from build123d import *

# Parameters (mm, degrees)
SKETCH_W           = 33
SKETCH_H           = 14
PAD_DEPTH          = 38
SKETCH001_W        = 4
SKETCH001_H        = 58.5
PAD001_DEPTH       = 33
SKETCH002_W        = 10
SKETCH002_H        = 4
PAD002_DEPTH       = 33
SKETCH003_W        = 32
SKETCH003_H        = 5
SKETCH003_H_2      = 9
SKETCH003_H_3      = 14
POCKET_DEPTH       = 12
POCKET_FACE14_W    = 33
POCKET_FACE14_H    = 38
POCKET_FACE14_W_2  = 32
POCKET_FACE14_H_2  = 5
POCKET_FACE14_H_3  = 9
POCKET_FACE14_H_4  = 14
POCKET001_DEPTH    = 2
SKETCH004_W        = 33
SKETCH004_H        = 38
SKETCH004_W_2      = 32
SKETCH004_H_2      = 4
SKETCH004_H_3      = 8
SKETCH004_H_4      = 13
PAD003_DEPTH       = 2
POCKET002_DEPTH    = 1
POCKET003_DEPTH    = 31.5
SKETCH006_W        = 14
SKETCH006_H        = 38
PAD004_DEPTH       = 1
PAD005_DEPTH       = 1
SKETCH007_W        = 37
SKETCH007_H        = 14
PAD006_DEPTH       = 2
SKETCH008_W        = 37
SKETCH008_H        = 2
PAD007_DEPTH       = 4
FILLET_R           = 4.74
FILLET001_R        = 4.74
FILLET002_R        = 1
FILLET003_R        = 1
FILLET004_R        = 1
FILLET005_R        = 1
FILLET005_FACE22_W = 18
FILLET005_FACE22_H = 2
PAD008_DEPTH       = 2
PAD008_FACE3_W     = 14
PAD008_FACE3_H     = 38
PAD009_DEPTH       = 2
PAD009_FACE3_W     = 18
PAD009_FACE3_H     = 2
PAD010_DEPTH       = 2
PAD010_FACE1_W     = 14
PAD010_FACE1_H     = 38
PAD011_DEPTH       = 2
SKETCH009_W        = 20
SKETCH009_H        = 11
POCKET004_DEPTH    = 38
FILLET006_R        = 5
FILLET007_R        = 1
FILLET008_R        = 1
SKETCH010_W        = 1
SKETCH010_H        = 0.5
PAD012_DEPTH       = 12


with BuildPart() as part:
    # Sketch → Pad (new body)
    with BuildSketch(Plane.XY):
        Rectangle(SKETCH_W, SKETCH_H)
    extrude(amount=PAD_DEPTH)

    # Sketch001 (on Face2 of Pad) → Pad001 (join)
    with BuildSketch(Plane.YZ.offset(16.5)):
        with Locations((-0.02597, 29.25)):
            Rectangle(SKETCH001_W, SKETCH001_H)
    extrude(amount=-PAD001_DEPTH)

    # Sketch002 (on Face9 of Pad001) → Pad002 (join)
    with BuildSketch(Plane.YZ.offset(16.5)):
        with Locations((0, 56.5)):
            Rectangle(SKETCH002_W, SKETCH002_H)
    extrude(amount=-PAD002_DEPTH)

    # Sketch003 (on Face4 of Pad002) → Pocket (cut)
    with BuildSketch(Plane(origin=(0, 7, 0), x_dir=(-1, 0, 0), z_dir=(0, 1, 0))):
        with Locations((0, 33.3)):
            Rectangle(SKETCH003_W, SKETCH003_H)
        with Locations((0, 23.9)):
            Rectangle(SKETCH003_W, SKETCH003_H_2)
        with Locations((0, 10)):
            Rectangle(SKETCH003_W, SKETCH003_H_3)
    extrude(amount=-POCKET_DEPTH, mode=Mode.SUBTRACT)

    # Pocket Face14 → Pocket001 (cut)
    with BuildSketch(Plane(origin=(0, 7, 19.929609), x_dir=(1, 0, 0), z_dir=(0, 1, 0))):
        with Locations((0, 0.929609)):
            Rectangle(POCKET_FACE14_W, POCKET_FACE14_H)
        with Locations((0, -13.370391)):
            Rectangle(POCKET_FACE14_W_2, POCKET_FACE14_H_2, mode=Mode.SUBTRACT)
        with Locations((0, -3.970391)):
            Rectangle(POCKET_FACE14_W_2, POCKET_FACE14_H_3, mode=Mode.SUBTRACT)
        with Locations((0, 9.929609)):
            Rectangle(POCKET_FACE14_W_2, POCKET_FACE14_H_4, mode=Mode.SUBTRACT)
    extrude(amount=-POCKET001_DEPTH, mode=Mode.SUBTRACT)

    # Sketch004 (on Face6 of Pocket001) → Pad003 (join)
    with BuildSketch(Plane(origin=(0, 5, 0), x_dir=(-1, 0, 0), z_dir=(0, 1, 0))):
        with Locations((0, 19)):
            Rectangle(SKETCH004_W, SKETCH004_H)
        with Locations((0, 33.8)):
            Rectangle(SKETCH004_W_2, SKETCH004_H_2, mode=Mode.SUBTRACT)
        with Locations((0, 24.4)):
            Rectangle(SKETCH004_W_2, SKETCH004_H_3, mode=Mode.SUBTRACT)
        with Locations((0, 10.5)):
            Rectangle(SKETCH004_W_2, SKETCH004_H_4, mode=Mode.SUBTRACT)
    extrude(amount=PAD003_DEPTH)

    # Pad003 Face14 → Pocket002 (cut)
    with BuildSketch(Plane(origin=(-16.5, -0.002687, 24.170063), x_dir=(0, 1, 0), z_dir=(-1, 0, 0))):
        Polygon((1.976717, -13.829937), (7.002687, -13.829937), (7.002687, 24.170063), (-6.997313, 24.170063), (-6.997313, -13.829937), (-2.023283, -13.829937), (-2.023283, -30.329937), (-4.997313, -30.329937), (-4.997313, -34.329937), (5.002687, -34.329937), (5.002687, -30.329937), (1.976717, -30.329937), align=None)
    extrude(amount=-POCKET002_DEPTH, mode=Mode.SUBTRACT)

    # Sketch005 (on Face4 of Pocket002) → Pocket003 (cut)
    with BuildSketch(Plane(origin=(-15.5, 0, 0), x_dir=(0, -1, 0), z_dir=(-1, 0, 0))):
        Polygon((-5, 3), (-5, 4), (-6, 4), align=None)
        Polygon((-5, 19.4), (-5, 20.4), (-6, 20.4), align=None)
        Polygon((-5, 30.8), (-5, 31.8), (-6, 31.8), align=None)
    extrude(amount=-POCKET003_DEPTH, mode=Mode.SUBTRACT)

    # Sketch006 (on Face4 of Pocket003) → Pad004 (join)
    with BuildSketch(Plane(origin=(-15.5, 0, 0), x_dir=(0, -1, 0), z_dir=(-1, 0, 0))):
        with Locations((0, 19)):
            Rectangle(SKETCH006_W, SKETCH006_H)
    extrude(amount=PAD004_DEPTH)

    # Pad004 Face9 → Pad005 (add)
    with BuildSketch(Plane(origin=(-15.5, -0.01617, 50.117925), x_dir=(0, 1, 0), z_dir=(-1, 0, 0))):
        Polygon((1.9902, -4.382075), (1.9902, 12.117925), (-2.0098, 12.117925), (-2.0098, -4.382075), (-4.98383, -4.382075), (-4.98383, -8.382075), (5.01617, -8.382075), (5.01617, -4.382075), align=None)
    extrude(amount=PAD005_DEPTH)

    # Sketch007 (on Face5 of Pad005) → Pad006 (join)
    with BuildSketch(Plane.XY.offset(38)):
        Rectangle(SKETCH007_W, SKETCH007_H)
    extrude(amount=PAD006_DEPTH)

    # Sketch008 (on Face19 of Pad006) → Pad007 (join)
    with BuildSketch(Plane(origin=(0, 7, 0), x_dir=(-1, 0, 0), z_dir=(0, 1, 0))):
        with Locations((0, 39)):
            Rectangle(SKETCH008_W, SKETCH008_H)
    extrude(amount=PAD007_DEPTH)

    # Fillet
    fillet_edges = [part.edges().sort_by_distance(p)[0] for p in [
        (0, -2.02597, 40),
    ]]
    fillet(fillet_edges, radius=FILLET_R)

    # Fillet001
    fillet001_edges = [part.edges().sort_by_distance(p)[0] for p in [
        (0, 1.97403, 40),
    ]]
    fillet(fillet001_edges, radius=FILLET001_R)

    # Fillet002
    fillet002_edges = [part.edges().sort_by_distance(p)[0] for p in [
        (0, -2.02597, 54.5),
    ]]
    fillet(fillet002_edges, radius=FILLET002_R)

    # Fillet003
    fillet003_edges = [part.edges().sort_by_distance(p)[0] for p in [
        (0, 1.97403, 54.5),
    ]]
    fillet(fillet003_edges, radius=FILLET003_R)

    # Fillet004
    fillet004_edges = [part.edges().sort_by_distance(p)[0] for p in [
        (0, 5, 54.5),
        (0, 5, 58.5),
    ]]
    fillet(fillet004_edges, radius=FILLET004_R)

    # Fillet005
    fillet005_edges = [part.edges().sort_by_distance(p)[0] for p in [
        (0, -5, 58.5),
        (0, -5, 54.5),
    ]]
    fillet(fillet005_edges, radius=FILLET005_R)

    # Fillet005 Face22 → Pad008 (add)
    with BuildSketch(Plane(origin=(-18.5, 2, 39), x_dir=(0, 1, 0), z_dir=(-1, 0, 0))):
        Rectangle(FILLET005_FACE22_W, FILLET005_FACE22_H)
    extrude(amount=PAD008_DEPTH)

    # Pad008 Face3 → Pad009 (add)
    with BuildSketch(Plane(origin=(-16.5, 0, 19), x_dir=(0, 1, 0), z_dir=(-1, 0, 0))):
        Rectangle(PAD008_FACE3_W, PAD008_FACE3_H)
    extrude(amount=PAD009_DEPTH)

    # Pad009 Face3 → Pad010 (add)
    with BuildSketch(Plane(origin=(18.5, 2, 39), x_dir=(0, -1, 0), z_dir=(1, 0, 0))):
        Rectangle(PAD009_FACE3_W, PAD009_FACE3_H)
    extrude(amount=PAD010_DEPTH)

    # Pad010 Face1 → Pad011 (add)
    with BuildSketch(Plane(origin=(16.5, 0, 19), x_dir=(0, -1, 0), z_dir=(1, 0, 0))):
        Rectangle(PAD010_FACE1_W, PAD010_FACE1_H)
    extrude(amount=PAD011_DEPTH)

    # Sketch009 (on Face47 of Pad011) → Pocket004 (cut)
    with BuildSketch(Plane(origin=(0, 0, 0), x_dir=(1, 0, 0), z_dir=(0, 0, -1))):
        with Locations((0, -1.5)):
            Rectangle(SKETCH009_W, SKETCH009_H)
    extrude(amount=-POCKET004_DEPTH, mode=Mode.SUBTRACT)

    # Fillet006
    fillet006_edges = [part.edges().sort_by_distance(p)[0] for p in [
        (-10, -4, 36.9),
        (-10, -4, 29.6),
        (-10, -4, 18.2),
        (-10, -4, 1.5),
        (10, -4, 36.9),
        (10, -4, 29.6),
        (10, -4, 18.2),
        (10, -4, 1.5),
    ]]
    fillet(fillet006_edges, radius=FILLET006_R)

    # Fillet007
    fillet007_edges = [part.edges().sort_by_distance(p)[0] for p in [
        (-10, 7, 36.9),
        (-10, 7, 30.1),
        (-10, 7, 18.7),
        (-10, 7, 2),
        (10, 7, 36.9),
        (10, 7, 30.1),
        (10, 7, 18.7),
        (10, 7, 2),
    ]]
    fillet(fillet007_edges, radius=FILLET007_R)

    # Fillet008
    fillet008_edges = [part.edges().sort_by_distance(p)[0] for p in [
        (18.5, 7, 19),
        (-18.5, 7, 19),
    ]]
    fillet(fillet008_edges, radius=FILLET008_R)

    # Sketch010 (on Face53 of Fillet008) → Pad012 (join)
    with BuildSketch(Plane(origin=(0, -5, 0), x_dir=(-1, 0, 0), z_dir=(0, 1, 0))):
        with Locations((-14, 31.05)):
            Rectangle(SKETCH010_W, SKETCH010_H)
        with Locations((14, 3.25)):
            Rectangle(SKETCH010_W, SKETCH010_H)
        with Locations((12, 3.25)):
            Rectangle(SKETCH010_W, SKETCH010_H)
        with Locations((-12, 3.25)):
            Rectangle(SKETCH010_W, SKETCH010_H)
        with Locations((-14, 3.25)):
            Rectangle(SKETCH010_W, SKETCH010_H)
        with Locations((-14, 19.65)):
            Rectangle(SKETCH010_W, SKETCH010_H)
        with Locations((14, 19.65)):
            Rectangle(SKETCH010_W, SKETCH010_H)
        with Locations((12, 19.65)):
            Rectangle(SKETCH010_W, SKETCH010_H)
        with Locations((-12, 19.65)):
            Rectangle(SKETCH010_W, SKETCH010_H)
        with Locations((-12, 31.05)):
            Rectangle(SKETCH010_W, SKETCH010_H)
        with Locations((12, 31.05)):
            Rectangle(SKETCH010_W, SKETCH010_H)
        with Locations((14, 31.05)):
            Rectangle(SKETCH010_W, SKETCH010_H)
    extrude(amount=PAD012_DEPTH)


solid = part.part
Check sheet for the modelled part. Datum: model origin and axes. Units: mm. A direction names the side the tool comes from. Round coordinates to 2 decimals unless told otherwise and drop trailing zeros. Loops run counter-clockwise (first coordinate to the right, second up) from the corner with the lowest first, then second, coordinate; pieces in that order, holes last. Notation, with made-up numbers: (-6.75, 74) -> (15.25, 74) arc R17 cw to (15.25, 85) -> close; hole circle Ø2 at (46, -3). An arc over 180 degrees is marked (long way). Put each result on its own line as item: value. Start each with the question number.
1. Scan lines: probe 1 along Z at (x, y) = (-10.5, -0.5); probe 2 along X at (y, z) = (3, 34); probe 3 along X at (y, z) = (0.75, 36). Record each from-to range of solid material in increasing order.
2. Access from +Z, -Z, +X, -X, +Y, -Y to the whole of each face (thin tool, end or side, straight path). Record for faces 5 (the face through (0.1, -4.4, 19.4)), 6 (the face through (0, 1.974, 49)), 7 (the face through (-10, 4, 37)).
3. Section check D-D (z = 46). Enter the section's corners in (x, y).
4. Section check B-B (z = 33). Enter the section's corners in (x, y), plus the area to 3 significant figures.
5. Draft check along Z on faces 1 (the face through (0, 8, 40)), 2 (the face through (-0.23, 3.4, 41.35)), 3 (the face through (-5, 4, 38)), 4 (the face through (0, -5, 56)). Enter one of: +Z half, -Z half, draft (parallel to the pull), parting line (faces both ways), or undercut.
6. Gauge pin test, flat ends, axial feed: pin 1 (3 mm diameter, centred on y = 4.5, z = 16.5, fed in from -X); pin 2 (1 mm diameter, centred on y = 4, z = 18.5, fed in from +X); pin 3 (6 mm diameter, centred on x = -1.5, y = 0, fed in from -Z). Record the tip position at first contact, or that the pin passes through.
Findings:
1. probe 1: z = 0 to 3, 17 to 19.4, 28.4 to 30.8, 35.8 to 58.5
1. probe 2: x = -18.5 to -15.5, 16 to 18.5
1. probe 3: x = -18.5 to -9.99, 9.99 to 18.5
2. face 5: none
2. face 6: +X, -X, +Y
2. face 7: -Z, +Y
3. outline: (-16.5, -2.03) -> (16.5, -2.03) -> (16.5, 1.97) -> (-16.5, 1.97) -> close
4. outline: (-18.5, -7) -> (18.5, -7) -> (18.5, 6) arc R1 ccw to (17.5, 7) -> (16, 7) -> (16, -5) -> (-15.5, -5) -> (-15.5, 7) -> (-17.5, 7) arc R1 ccw to (-18.5, 6) -> close
4. area: 140 mm^2
5. face 1: +Z half
5. face 2: undercut
5. face 3: -Z half
5. face 4: draft
6. pin 1: stops at x = -18.5
6. pin 2: stops at x = 18.5
6. pin 3: stops at z = 38
